Design review of the part built by this model. Coordinates are the model's own, in mm. A direction names the side the tool comes from. Give positions to 0.01 mm unless a question says otherwise; leave off trailing zeros. Loops run counter-clockwise (first coordinate to the right, second up) from the corner with the lowest first, then second, coordinate; pieces in that order, holes last. Notation, with made-up numbers: (15, 54.25) -> (21, 54.25) arc R14 ccw to (21, 63.25) -> close; hole circle Ø2 at (14, -1.75). An arc over 180 degrees is marked (long way). Use a Markdown table: item, result. Add a question column.
1. For pin 1 Ø1.8 at (x, y) = (-5, 1.5) entering from -Z, flat-tipped, find the tip position at first contact; note if it passes through.
2. To check wall thickness, follow line 1 (Y direction, x = 5, z = 18); line 2 (X direction, y = 0.9, z = -12); line 3 (Z direction, x = -1, y = 5.6). State the ranges of each line that lie inside material, in increasing order.
3. Add section A-A (x = -5). State the section outline as (y, z) points, and give its area (3 significant figures).
4. Add section C-C (z = 18.5). State the section outline as (x, y) points.
5. For faces 4 (the flat face through (0, 6, 15)), 5 (the flat face through (11, 3, -5)), list the 3-axis set-ups (+Z, -Z, +X, -X, +Y, -Y) from which the entire face can be reached by the end or side of a thin tool; tool diameter is ignored.
6. Add section D-D (y = 3). State the section outline as (x, z) points, and give its area (3 significant figures).
7. Add section B-B (z = 9.5). State the section outline as (x, y) points.
8. Draft analysis for pull direction X (two halves, no side actions). For faces 1 (the flat face through (0, 0, 15)), 2 (the cylindrical face through (-11.92, 2.39, 0.32)), 3 (the cylindrical face through (-17.53, 5.4, -0.32)), state which applies: pulls with the +X half, pulls with the -X half, needs draft (parallel to the pull), parting line crosses it, or undercut.
```python
from build123d import *

# Parameters (mm, degrees)
SKETCH1_W           = 36.2
SKETCH1_H           = 45
BOSS_EXTRUDE1_DEPTH = 6
SKETCH2_R           = 1.6
CUT_EXTRUDE1_DEPTH  = 49.873407902
SKETCH4_W           = 22
SKETCH4_H           = 6
CUT_EXTRUDE2_DEPTH  = 35
FILLET1_R           = 2


with BuildPart() as part:
    # Sketch1 → Boss-Extrude1 (new body)
    with BuildSketch(Plane(origin=(0, 0, 0), x_dir=(1, 0, 0), z_dir=(0, 1, 0))):
        Rectangle(SKETCH1_W, SKETCH1_H)
    extrude(amount=BOSS_EXTRUDE1_DEPTH)

    # Sketch2 → Cut-Extrude1 (cut, through all)
    with BuildSketch(Plane.XY.offset(22.5)):
        with Locations((-5, 3)):
            Circle(SKETCH2_R)
        with Locations((-13.4, 3)):
            Circle(SKETCH2_R)
        with Locations((5, 3)):
            Circle(SKETCH2_R)
        with Locations((13.4, 3)):
            Circle(SKETCH2_R)
    extrude(amount=-CUT_EXTRUDE1_DEPTH, mode=Mode.SUBTRACT)

    # Sketch4 → Cut-Extrude2 (cut)
    with BuildSketch(Plane(origin=(0, 0, -22.5), x_dir=(-1, 0, 0), z_dir=(0, 0, -1))):
        with Locations((0, 3)):
            Rectangle(SKETCH4_W, SKETCH4_H)
    extrude(amount=-CUT_EXTRUDE2_DEPTH, mode=Mode.SUBTRACT)

    # Fillet1
    fillet1_edges = [part.edges().sort_by_distance(p)[0] for p in [
        (-18.1, 6, 0),
        (18.1, 6, 0),
    ]]
    fillet(fillet1_edges, radius=FILLET1_R)


solid = part.part
```
Taken from the geometry:
| question | item | result |
|---|---|---|
| 1 | pin 1 | stops at z = 12.5 |
| 2 | line 1 | y = 0 to 1.4, 4.6 to 6 |
| 2 | line 2 | x = -18.1 to -11, 11 to 18.1 |
| 2 | line 3 | z = 12.5 to 22.5 |
| 3 | outline | (0, 12.5) -> (1.4, 12.5) -> (1.4, 22.5) -> (0, 22.5) -> close; (4.6, 12.5) -> (6, 12.5) -> (6, 22.5) -> (4.6, 22.5) -> close |
| 3 | area | 28.0 mm^2 |
| 4 | outline | (-18.1, 0) -> (18.1, 0) -> (18.1, 4) arc R2 ccw to (16.1, 6) -> (-16.1, 6) arc R2 ccw to (-18.1, 4) -> close; hole circle Ø3.2 at (-13.4, 3); hole circle Ø3.2 at (-5, 3); hole circle Ø3.2 at (5, 3); hole circle Ø3.2 at (13.4, 3) |
| 5 | face 4 | +Z, -Z, +X, -X, +Y |
| 5 | face 5 | -Z, +Y, -Y |
| 6 | outline | (-18.1, -22.5) -> (-15, -22.5) -> (-15, 22.5) -> (-18.1, 22.5) -> close; (-11.8, -22.5) -> (-11, -22.5) -> (-11, 12.5) -> (-6.6, 12.5) -> (-6.6, 22.5) -> (-11.8, 22.5) -> close; (-3.4, 12.5) -> (3.4, 12.5) -> (3.4, 22.5) -> (-3.4, 22.5) -> close; (6.6, 12.5) -> (11, 12.5) -> (11, -22.5) -> (11.8, -22.5) -> (11.8, 22.5) -> (6.6, 22.5) -> close; (15, -22.5) -> (18.1, -22.5) -> (18.1, 22.5) -> (15, 22.5) -> close |
| 6 | area | 507 mm^2 |
| 7 | outline | (-18.1, 0) -> (-11, 0) -> (-11, 6) -> (-16.1, 6) arc R2 ccw to (-18.1, 4) -> close; (11, 0) -> (18.1, 0) -> (18.1, 4) arc R2 ccw to (16.1, 6) -> (11, 6) -> close; hole circle Ø3.2 at (-13.4, 3); hole circle Ø3.2 at (13.4, 3) |
| 8 | face 1 | needs draft |
| 8 | face 2 | undercut |
| 8 | face 3 | pulls with the -X half |
